Part print with two shaded views. Sizes in mm from the minimum x, y, z corner. A direction names the side the tool comes from. Give positions to 0.01 mm unless a question says otherwise; leave off trailing zeros. Order: outer loops, then holes, each group sorted by start corner. A loop starts at its lowest first (then second) coordinate and runs counter-clockwise, first axis right, second up. Notation, with made-up numbers: (83, -21.75) -> (125, -21.75) arc R11 cw to (125, -15.75) -> close; hole circle Ø4 at (-30, 39.5). An arc over 180 degrees is marked (long way). Write item = value, one per line. Start each with the question number.
Item 1: Flat gauge pins, fed straight in: P1, Ø2, axis at x = 9, y = 7, coming from the +Z side; P2, Ø2.5, axis at x = 4, y = 4.5, coming from the +Z side; P3, Ø1.5, axis at y = 8, z = 13.5, coming from the +X side. Where does each tip first touch, or does it go through?
Item 2: Pull direction Z, two halves, no side cores. Call the marked faces 1, 2 and 3: +Z half, -Z half, draft (parallel to the pull), parting line (faces both ways), or undercut.
Item 3: Band-saw the part on A-A on z = 4.25. Write the cut outline in (x, y), plus the area to 3 significant figures.
Item 4: Band-saw the part on C-C on y = 7.25. Write the cut outline in (x, z).
Item 5: Band-saw the part on B-B on x = 5. Write the cut outline in (y, z).
Item 6: Band-saw the part on D-D on x = 1.5. Write the cut outline in (y, z).
Item 7: Tool access for the marked faces 4 and 5: list every direction of +Z, -Z, +X, -X, +Y, -Y with a clear straight run to the whole face (end or side of a thin tool).
Item 8: Drill centre lines: line 1 along Z through (x, y) = (5, 7.6); line 2 along Y through (x, z) = (9.5, 5.5); line 3 along Z through (x, y) = (1.75, 4.5). Where is each one in solid material? Low to high.
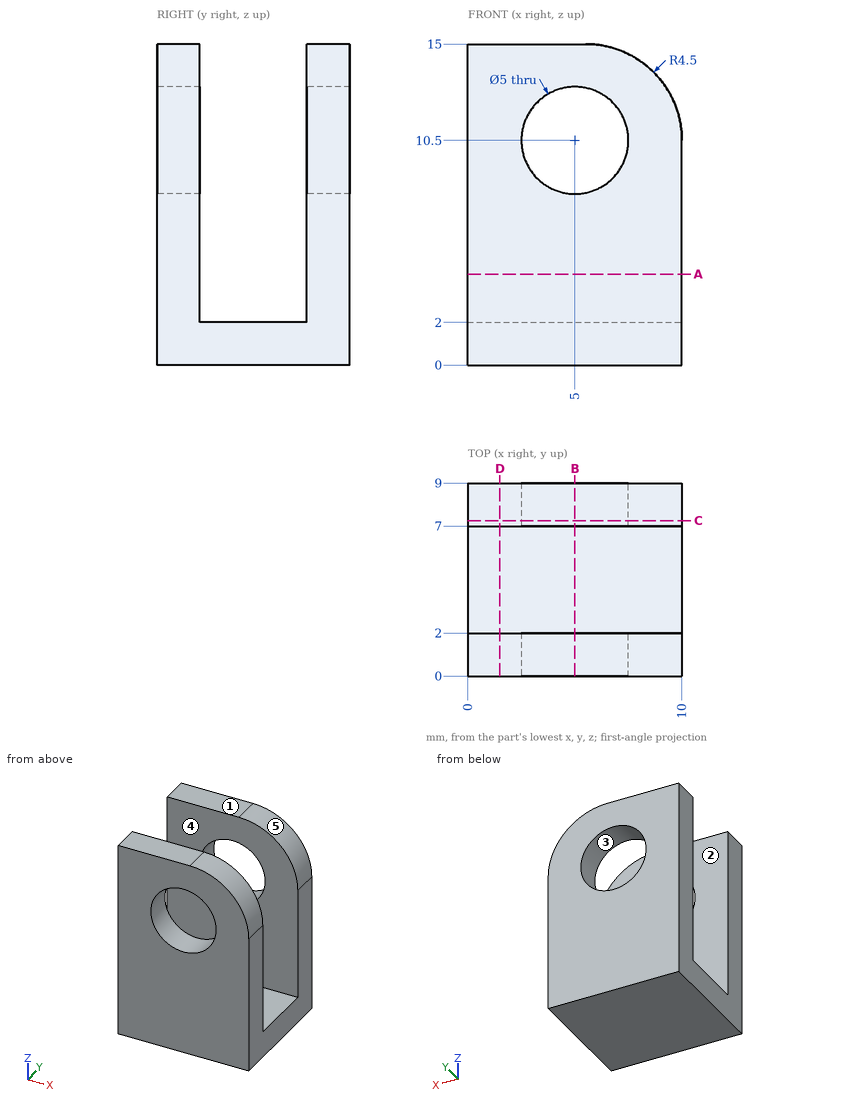
Values found:
q1.P1 = 14.24
q1.P2 = 2
q1.P3 = 9.4
q2.face_1 = +Z half
q2.face_2 = draft
q2.face_3 = undercut
q3.outline = (0, 0) -> (10, 0) -> (10, 2) -> (0, 2) -> close; (0, 7) -> (10, 7) -> (10, 9) -> (0, 9) -> close
q3.area = 40.0 mm^2
q4.outline = (0, 0) -> (10, 0) -> (10, 10.5) arc R4.5 ccw to (5.5, 15) -> (0, 15) -> close; hole circle Ø5 at (5, 10.5)
q5.outline = (0, 0) -> (9, 0) -> (9, 8) -> (7, 8) -> (7, 2) -> (2, 2) -> (2, 8) -> (0, 8) -> close; (0, 13) -> (2, 13) -> (2, 15) -> (0, 15) -> close; (7, 13) -> (9, 13) -> (9, 15) -> (7, 15) -> close
q6.outline = (0, 0) -> (9, 0) -> (9, 15) -> (7, 15) -> (7, 2) -> (2, 2) -> (2, 15) -> (0, 15) -> close
q7.face_4 = +Z, +X, -X
q7.face_5 = +Z, +X, +Y, -Y
q8.line_1 = 0 to 8, 13 to 15
q8.line_2 = 0 to 2, 7 to 9
q8.line_3 = 0 to 2
